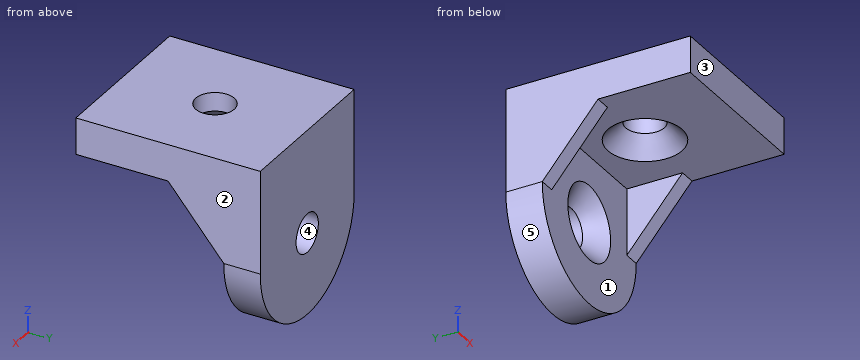
```python
from build123d import *

# Parameters (mm, degrees)
SKETCH_1_W      = 38
SKETCH_1_H      = 43
EXTRUDE_1_DEPTH = 8.5
EXTRUDE_2_DEPTH = 8.5
EXTRUDE_3_DEPTH = 3.8


with BuildPart() as part:
    # 草图1 → 凸台-拉伸1 (new body)
    with BuildSketch(Plane.XY):
        Rectangle(SKETCH_1_W, SKETCH_1_H)
    extrude(amount=EXTRUDE_1_DEPTH)

    # 草图2 → 凸台-拉伸2 (add)
    with BuildSketch(Plane(origin=(0, 21.5, 0), x_dir=(1, 0, 0), z_dir=(0, 1, 0))):
        with BuildLine():
            Line((-19, -8.5), (19, -8.5))
            Line((19, -8.5), (19, 15.5))
            ThreePointArc((19, 15.5), (0, 34.5), (-19, 15.5))
            Line((-19, 15.5), (-19, -8.5))
        make_face()
    extrude(amount=-EXTRUDE_2_DEPTH)

    # 草图5 → 凸台-拉伸3 (add)
    with BuildSketch(Plane(origin=(19, 0, 0), x_dir=(0, 0, -1), z_dir=(1, 0, 0))):
        Polygon((15.5, 13), (0, 13), (0, 0), align=None)
    extrude_3 = extrude(amount=-EXTRUDE_3_DEPTH)

    # 镜向1: 凸台-拉伸3 across plane
    add(extrude_3.mirror(Plane(origin=(0, 0, 0), x_dir=(0, 0, 1), z_dir=(1, 0, 0))))

    # 草图6 → M8 平锥沉头螺钉的锥形沉头孔1 (revolve, cut)
    with BuildSketch(Plane.YZ):
        Polygon((0, 0), (0, 8.5), (4.5, 8.5), (4.5, 4.15), (8.65, 0), align=None)
    revolve(axis=Axis((0, 0, -6.35), (0, 0, 1)), mode=Mode.SUBTRACT)

    # 草图8 → M8 平锥沉头螺钉的锥形沉头孔2 (revolve, cut)
    with BuildSketch(Plane(origin=(0, 13, -15.5), x_dir=(0, 0, -1), z_dir=(1, 0, 0))):
        Polygon((0, 0), (0, 8.5), (4.5, 8.5), (4.5, 4.15), (8.65, 0), align=None)
    revolve(axis=Axis((0, 6.65, -15.5), (0, 1, 0)), mode=Mode.SUBTRACT)


solid = part.part
```
Check sheet for the modelled part. Datum: model origin and axes. Units: mm. Face numbers are marked on the shaded views. A direction names the side the tool comes from. Round coordinates to 2 decimals unless told otherwise and drop trailing zeros. Write each loop counter-clockwise with the first axis right and the second up, starting at its lowest first coordinate (ties: lowest second). Pieces come first, ordered by that corner, then holes. Notation, with made-up numbers: (-39, -11.5) -> (-18, -11.5) arc R13 cw to (-18, -0.5) -> close; hole circle Ø10 at (-16, 80). An arc over 180 degrees is marked (long way). Put each result on its own line as item: value.
(1) Sectioned sample at A-A (x = 0). Enter the section's corners in (y, z).
Values found:
outline: (-21.5, 0) -> (-8.65, 0) -> (-4.5, 4.15) -> (-4.5, 8.5) -> (-21.5, 8.5) -> close; (4.5, 4.15) -> (8.65, 0) -> (13, 0) -> (13, -6.85) -> (17.15, -11) -> (21.5, -11) -> (21.5, 8.5) -> (4.5, 8.5) -> close; (13, -34.5) -> (21.5, -34.5) -> (21.5, -20) -> (17.15, -20) -> (13, -24.15) -> close
(2) Sectioned sample at B-B (z = 2.5). Enter the section's corners in (x, y), plus the area to 3 significant figures.
Values found:
outline: (-19, -21.5) -> (19, -21.5) -> (19, 21.5) -> (-19, 21.5) -> close; hole circle Ø12.3 at (0, 0)
area: 1,520 mm^2
(3) Material ranges on line 1 (Y direction, x = 0, z = 5.75); line 2 (Z direction, x = 0, y = 19.5); line 3 (Z direction, x = 12, y = 1), recorded low to high.
Values found:
line 1: y = -21.5 to -4.5, 4.5 to 21.5
line 2: z = -34.5 to -20, -11 to 8.5
line 3: z = 0 to 8.5
(4) Sectioned sample at C-C (y = -16). Enter the section's corners in (x, z), plus the area to 3 significant figures.
Values found:
outline: (-19, 0) -> (19, 0) -> (19, 8.5) -> (-19, 8.5) -> close
area: 323 mm^2
(5) Mould release check, pull along X, two halves, no side actions. Record for the marked faces 3, 4 and 5: released by +X, released by -X, zero draft, split by the parting line, or undercut.
Values found:
face 3: zero draft
face 4: undercut
face 5: split by the parting line
(6) Go/stop test with flat-tipped pins: pin 1 Ø17 at (x, y) = (-2.5, 3.5) entering from -Z; pin 2 Ø10.5 at (x, y) = (0, 0) entering from -Z; pin 3 Ø4 at (x, z) = (-1, -26) entering from -Y. Record where each tip stops, or that it passes through.
Values found:
pin 1: stops at z = 0
pin 2: stops at z = 3.4
pin 3: stops at y = 13
(7) Sectioned sample at D-D (x = -13.5). Enter the section's corners in (y, z).
Values found:
outline: (-21.5, 0) -> (13, 0) -> (13, -28.87) -> (21.5, -28.87) -> (21.5, 8.5) -> (-21.5, 8.5) -> close
(8) Tool access check on the marked faces 1 and 2. Record the directions out of +Z, -Z, +X, -X, +Y, -Y that give a thin tool (end or side, any length) a straight path to the whole face; none if there is none.
Values found:
face 1: -Z, -Y
face 2: +Z, -Z, +X, +Y, -Y
